Autodesk Inventor part; units mm, degrees
ref_plane "YZ Plane" through (0, 0, 0) normal (1, 0, 0) x (0, 1, 0)
ref_plane "XZ Plane" through (0, 0, 0) normal (0, 1, 0) x (-1, 0, 0)
ref_plane "XY Plane" through (0, 0, 0) normal (0, 0, 1) x (1, 0, 0)
sketch "Sketch1" plane through (0, 0, 0) normal (0, 0, 1) x (1, 0, 0)
  circle A0 centre (0, 0) radius 22.225
  circle A1 centre (0, 0) radius 17.225
  line L0 (-17.225, -2) -> (17.225, -2)
  line L1 (17.225, -2) -> (17.225, 2)
  line L2 (17.225, 2) -> (-17.225, 2)
  line L3 (-17.225, 2) -> (-17.225, -2)
  line L4 (-17.225, -2) -> (17.225, 2) construction
  line L5 (17.225, -2) -> (-17.225, 2) construction
  dimension "d0" = 44.45
  dimension "d1" = 34.45
  dimension "d2" = 4
extrude "Extrusion1" add sketch "Sketch1" against normal blind 4 contours A0 | A1 L0 L2 | L1 L0 A1 | A1 L2 L1 | L2 A1 | A1 L0 | A1 L3 L2 | L0 L3 A1
extrude "Extrusion2" add sketch "Sketch1" along normal blind 20 contours A1 L0 L2 | L2 A1 | A1 L0
extrude "Extrusion3" cut sketch "Sketch1" along normal blind 4 contours A1 L0 L2 | L1 L0 A1 | A1 L2 L1 | A1 L3 L2 | L0 L3 A1
equation "\"d0\" = tube_ID"
equation "\"d3\" = sheet"
equation "\"d5\" = 5 * sheet"
equation "\"d7\" = sheet"
properties part number "battery_endcap"
Verification items for the finished model (mm, model axes). A direction names the side the tool comes from. Give positions to 0.01 mm unless a question says otherwise; leave off trailing zeros. Write each loop counter-clockwise with the first axis right and the second up, starting at its lowest first coordinate (ties: lowest second). Pieces come first, ordered by that corner, then holes. Notation, with made-up numbers: M 53,-16.5 L 65,-16.5 A27 cw 65,1.5 Z; hole C -34.75,-12 d3. An arc over 180 degrees is marked long. Put each result on its own line as item: value. Start each with the question number.
1. Scan lines: line 1 along Z through (x, y) = (15.5, -12.5); line 2 along X through (y, z) = (0.5, 10); line 3 along Y through (x, z) = (-10.5, -3). Record each from-to range of solid material in increasing order. Write a range as [from, to].
2. Set-up check for faces 1 (the face through (0, 0, 4)), 2 (the face through (0, 0, 0)), 3 (the face through (0, 0, 20)): record each of +Z, -Z, +X, -X, +Y, -Y from which the full face is reachable in a straight line by a thin tool's end or side.
3. Section check B-B (x = 0). Record the cut outline in (y, z) (3 decimals), and give its area (3 significant figures).
4. Draft check along Y on faces 4 (the face through (0, 0, -4)), 5 (the face through (15.91, 6.6, 9.86)), 6 (the face through (0, -2, 2)). Enter one of: +Y half, -Y half, draft (parallel to the pull), parting line (faces both ways), or undercut.
5. Section check A-A (y = 0). Record the cut outline in (x, z) (3 decimals).
6. Section check C-C (x = -6.5). Record the cut outline in (y, z).
7. Go/stop test with flat-tipped pins: pin 1 Ø3 at (x, z) = (-2, 2) entering from +Y; pin 2 Ø6 at (y, z) = (16, 16) entering from +X; pin 3 Ø3 at (x, z) = (11, 14) entering from -Y. Record where each tip stops, or that it passes through.
8. Section check D-D (z = 16.5). Record the cut outline in (x, y) (3 decimals), and give its area (3 significant figures).
Answer list:
1. line 1: [-4, 0]
1. line 2: [-17.22, 17.22]
1. line 3: [-19.59, 19.59]
2. face 1: +X, -X
2. face 2: none
2. face 3: +Z, +X, -X, +Y, -Y
3. outline: M -22.225,-4 L 22.225,-4 L 22.225,0 L 17.225,0 L 17.225,20 L -17.225,20 L -17.225,0 L -22.225,0 Z; hole M -2,0 L 2,0 L 2,4 L -2,4 Z
3. area: 851 mm2
4. face 4: draft
4. face 5: parting line
4. face 6: undercut
5. outline: M -22.225,-4 L 22.225,-4 L 22.225,0 L -22.225,0 Z; M -17.225,4 L 17.225,4 L 17.225,20 L -17.225,20 Z
6. outline: M -21.25,-4 L 21.25,-4 L 21.25,0 L 15.95,0 L 15.95,20 L -15.95,20 L -15.95,0 L -21.25,0 Z; hole M -2,0 L 2,0 L 2,4 L -2,4 Z
7. pin 1: y = 17.22
7. pin 2: x = 11.3
7. pin 3: y = -14.37
8. outline: C 0,0 d34.45
8. area: 932 mm2
